Geometry check sheet. Reference: the model listing, model coordinates, mm. Round coordinates to 2 decimals unless told otherwise and drop trailing zeros. Write each loop counter-clockwise with the first axis right and the second up, starting at its lowest first coordinate (ties: lowest second). Pieces come first, ordered by that corner, then holes. Notation, with made-up numbers: (47, 13.25) -> (84, 13.25) arc R29 ccw to (84, 38.25) -> close; hole circle Ø5 at (4, 42.25). An arc over 180 degrees is marked (long way). Return JSON: item names as keys, results as strings. Group by question number.
from build123d import *

# Parameters (mm, degrees)
F0_W = 76
F0_H = 3.75


with BuildPart() as f1:
    # F0 (on Top) → F1 (revolve)
    with BuildSketch(Plane.XY):
        Polygon((-63.5, 0), (-38, 0), (-38, 3.75), (-38, 4), (-63.5, 4), align=None)
        with Locations((0, 1.875)):
            Rectangle(F0_W, F0_H)
        Polygon((38, 0), (63.5, 0), (63.5, 4), (38, 4), (38, 3.75), align=None)
    revolve(axis=Axis((0, 0, 0), (1, 0, 0)))


solid = f1.part
1) Sectioned sample at C-C on x = 55. Enter the section's corners in (y, z).
2) Mould release check, pull along X, two halves, no side actions. Record for faces 1 (the face through (-50.928, -0.867, -3.905)), 2 (the face through (0.532, -3.746, 0.165)), 3 (the face through (63.5, 0, 0)), 4 (the face through (-63.5, 0, 0)): +X half, -X half, draft (parallel to the pull), parting line (faces both ways), or undercut.
3) Material ranges on probe 1 along X at (y, z) = (-3.5, 1.5); probe 2 along Z at (x, y) = (-10, -0.25); probe 3 along Z at (x, y) = (-55, 0.25), recorded low to high. Write a range as [from, to].
4) Sectioned sample at D-D on x = -20. Enter the section's corners in (y, z).
5) Sectioned sample at A-A on y = 0. Enter the section's corners in (x, z).
6) Go/stop test with flat-tipped pins: P1, Ø2, axis at x = 4, z = 0, coming from the +Y side; P2, Ø3, axis at x = 33, y = 3, coming from the -Z side; P3, Ø2, axis at x = -23, y = -1, coming from the -Z side. Record where each tip stops, or that it passes through.
Evaluation:
{
 "1": {"outline": "circle Ø8 at (0, 0)"},
 "2": {"face 1": "draft", "face 2": "undercut", "face 3": "+X half", "face 4": "-X half"},
 "3": {"probe 1": "x = [-63.5, -38], [38, 63.5]", "probe 2": "z = [-3.74, 3.74]", "probe 3": "z = [-3.99, 3.99]"},
 "4": {"outline": "circle Ø7.5 at (0, 0)"},
 "5": {"outline": "(-63.5, -4) -> (-38, -4) -> (-38, -3.75) -> (38, -3.75) -> (38, -4) -> (63.5, -4) -> (63.5, 4) -> (38, 4) -> (38, 3.75) -> (-38, 3.75) -> (-38, 4) -> (-63.5, 4) -> close"},
 "6": {"P1": "stops at y = 3.75", "P2": "stops at z = -3.44", "P3": "stops at z = -3.75"}
}
